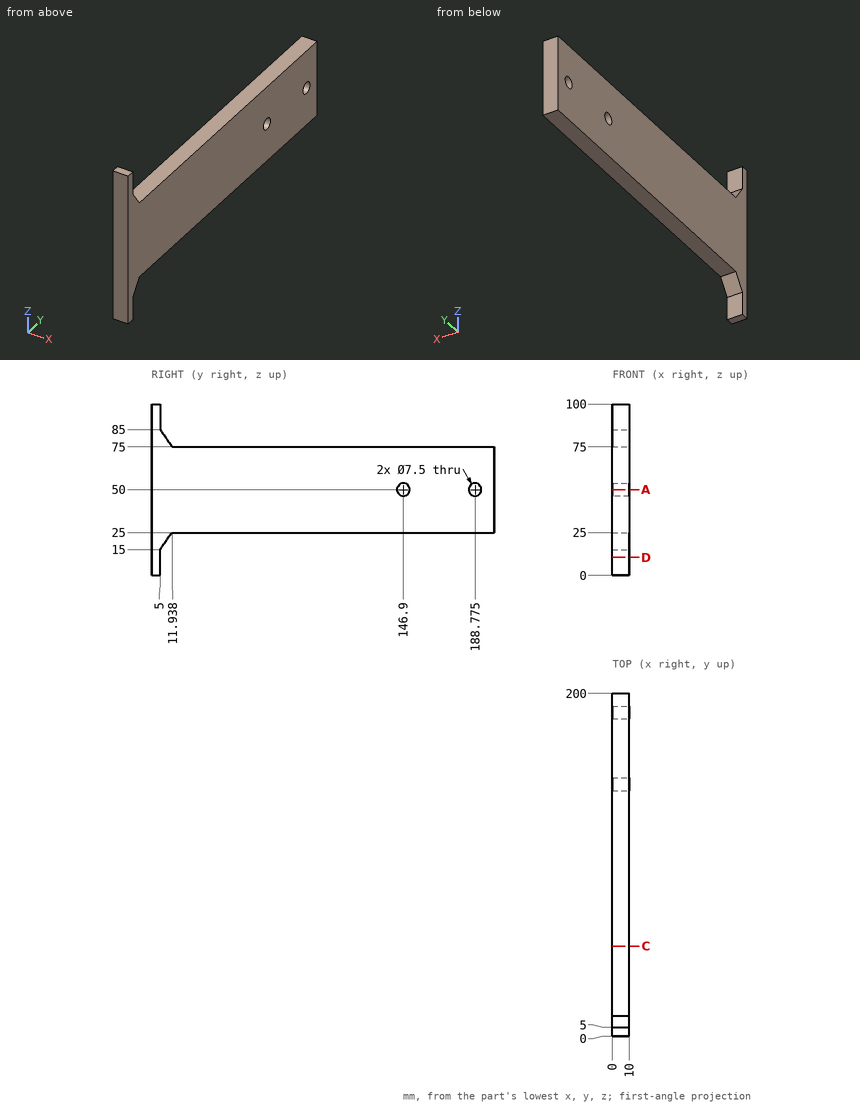
Drawing for the job (mm, zero at the part's lowest x, y, z). Coordinates: 2 decimals unless noted, no trailing zeros. Write each loop counter-clockwise with the first axis right and the second up, starting at its lowest first coordinate (ties: lowest second). Pieces come first, ordered by that corner, then holes. Notation, with made-up numbers: (3, 51) -> (40, 51) arc R9 ccw to (40, 56) -> close; hole circle Ø10 at (65.5, -25). An arc over 180 degrees is marked (long way). One line per item, written item: value. Start each with the question number.
1) Probe probe 1 along Z at (x, y) = (2, 22); probe 2 along Z at (x, y) = (8.5, 146.5); probe 3 along Y at (x, z) = (5.25, 13.5). List the from-to ranges inside material, lowest first.
2) Slice it at C-C on y = 52.5. Write the cut outline in (x, z).
3) Flat gauge pins, fed straight in: pin 1 Ø3 at (x, z) = (5.5, 9) entering from +Y; pin 2 Ø6 at (x, y) = (8.5, 28.5) entering from -Z; pin 3 Ø4 at (x, z) = (2.5, 55) entering from -Y; pin 4 Ø3 at (x, z) = (4, 82.5) entering from +Y (1 decimal). Where does each tip first touch, or does it go through?
4) Slice it at D-D on z = 10.5. Write the cut outline in (x, y).
5) Slice it at A-A on z = 50. Count the separate pieces of the cut face and the enclosed holes in it, then the cut area to 3 significant figures.
Answers follow:
1. probe 1: 25 to 75
1. probe 2: 25 to 46.27, 53.73 to 75
1. probe 3: 0 to 5
2. outline: (0, 25) -> (10, 25) -> (10, 75) -> (0, 75) -> close
3. pin 1: y = 5
3. pin 2: z = 25
3. pin 3: y = 0
3. pin 4: y = 7.8
4. outline: (0, 0) -> (10, 0) -> (10, 5) -> (0, 5) -> close
5. separate pieces: 3
5. enclosed holes: 0
5. area: 1,850 mm2
